```python
from build123d import *

# Parameters (mm, degrees)
SKETCH1_W                  = 20
SKETCH1_H                  = 37.5
SKETCH1_W_2                = 192
SKETCH1_H_2                = 30
BOSS_EXTRUDE1_DEPTH        = 10
F_4_0_209_DIAMETER_HOLE1_D = 5.3086
SKETCH6_W                  = 15
SKETCH6_H                  = 30
BOSS_EXTRUDE2_DEPTH        = 30
BOSS_EXTRUDE3_START        = 30
SKETCH6_3_W                = 100
SKETCH6_3_H                = 30
SKETCH6_3_W_2              = 15
BOSS_EXTRUDE3_DEPTH        = 15
FILLET2_R                  = 7


with BuildPart() as part:
    # Sketch1 → Boss-Extrude1 (new body)
    with BuildSketch(Plane.XY):
        with Locations((-86, 33.75)):
            Rectangle(SKETCH1_W, SKETCH1_H)
        Rectangle(SKETCH1_W_2, SKETCH1_H_2)
        with Locations((-86, -33.75)):
            Rectangle(SKETCH1_W, SKETCH1_H)
        with Locations((86, -33.75)):
            Rectangle(SKETCH1_W, SKETCH1_H)
        with Locations((86, 33.75)):
            Rectangle(SKETCH1_W, SKETCH1_H)
    extrude(amount=BOSS_EXTRUDE1_DEPTH)

    # #4 (0.209) Diameter Hole1 (through all)
    with Locations(Plane.XY.offset(10)):
        with Locations((-86, 42.5), (-86, -42.5), (86, -42.5), (86, 42.5)):
            Hole(F_4_0_209_DIAMETER_HOLE1_D / 2)

    # Sketch6 → Boss-Extrude2 (add)
    with BuildSketch(Plane.XY.offset(10)):
        with Locations((-57.5, 0)):
            Rectangle(SKETCH6_W, SKETCH6_H)
        with Locations((57.5, 0)):
            Rectangle(SKETCH6_W, SKETCH6_H)
    extrude(amount=BOSS_EXTRUDE2_DEPTH)

    # Sketch6<3> → Boss-Extrude3 (add)
    with BuildSketch(Plane.XY.offset(10).offset(BOSS_EXTRUDE3_START)):
        Rectangle(SKETCH6_3_W, SKETCH6_3_H)
        with Locations((-57.5, 0)):
            Rectangle(SKETCH6_3_W_2, SKETCH6_3_H)
        with Locations((57.5, 0)):
            Rectangle(SKETCH6_3_W_2, SKETCH6_3_H)
    extrude(amount=BOSS_EXTRUDE3_DEPTH)

    # Fillet2
    fillet2_edges = [part.edges().sort_by_distance(p)[0] for p in [
        (0, 15, 40),
        (0, -15, 40),
        (0, 15, 55),
        (-65, 0, 55),
        (0, -15, 55),
        (65, 0, 55),
        (-70.5, -15, 10),
        (-70.5, 15, 10),
        (0, -15, 10),
        (70.5, -15, 10),
        (0, 15, 10),
        (70.5, 15, 10),
        (-50, 15, 25),
        (-65, 0, 10),
        (-65, 15, 32.5),
        (-65, -15, 32.5),
        (-50, -15, 25),
        (-50, 0, 10),
        (65, -15, 32.5),
        (65, 15, 32.5),
        (50, 0, 10),
        (50, 15, 25),
        (50, -15, 25),
        (65, 0, 10),
    ]]
    fillet(fillet2_edges, radius=FILLET2_R)


solid = part.part
```
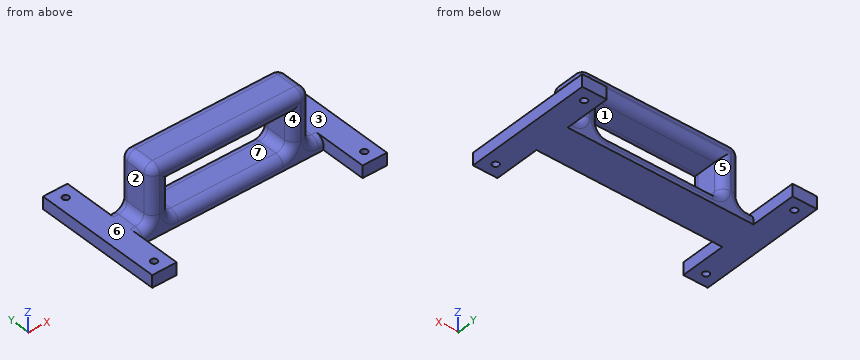
Work out the finished part from the listing and answer in its coordinate system (mm). Face numbers are marked on the shaded views. A direction names the side the tool comes from. Give positions to 0.01 mm unless a question says otherwise; leave off trailing zeros. Order: outer loops, then holes, each group sorted by start corner. A loop starts at its lowest first (then second) coordinate and runs counter-clockwise, first axis right, second up. Notation, with made-up numbers: (27.25, 65.5) - (70.25, 65.5) arc R20 cw to (70.25, 98.5) - close; hole circle Ø7 at (30.5, -28). An arc over 180 degrees is marked (long way). One line per item, written item: value. Start each with the question number.
1. Section A-A, the plane z = 34 is taken. Write down the section's boundary in (x, y).
2. Section C-C, the plane y = -23 is taken. Write down the section's boundary in (x, z), then the cut area to 3 significant figures.
3. Which of the six approach directions +Z, -Z, +X, -X, +Y, -Y give full straight-line access (tool end or side, diameter ignored) to the marked faces 4, 5, 6 and 7?
4. Section B-B, the plane x = -86 is taken. Write down the section's boundary in (y, z).
5. For a pull along Z with two mould halves and no side action, classify the marked faces 1, 2 and 3 as released by +Z, released by -Z, zero draft, split by the parting line, or undercut.
6. Consider line 1 (Y direction, x = 86, z = 5); line 2 (X direction, y = 34.5, z = 6.5); line 3 (X direction, y = 42, z = 3). Determine where each line is inside the solid, lowest interval first.
7. Section D-D, the plane x = -32 is taken. Write down the section's boundary in (y, z).
8. Each of these flat-tipped pins is pushed along its axis until it touches: pin 1 Ø8 at (y, z) = (2, 30) entering from -X; pin 2 Ø6 at (x, y) = (-86, -42.5) entering from +Z; pin 3 Ø17.5 at (y, z) = (-2.5, 33.5) entering from +X. Where does it stop, or does it pass through?
Filled sheet:
1. outline: (-65, -8) arc R7 ccw to (-58, -15) - (-57, -15) arc R7 ccw to (-50, -8) - (-50, 8) arc R7 ccw to (-57, 15) - (-58, 15) arc R7 ccw to (-65, 8) - close; (50, -8) arc R7 ccw to (57, -15) - (58, -15) arc R7 ccw to (65, -8) - (65, 8) arc R7 ccw to (58, 15) - (57, 15) arc R7 ccw to (50, 8) - close
2. outline: (-96, 0) - (-76, 0) - (-76, 10) - (-96, 10) - close; (76, 0) - (96, 0) - (96, 10) - (76, 10) - close
2. area: 400 mm²
3. face 4: -Y
3. face 5: +Y
3. face 6: +Z, -X, +Y, -Y
3. face 7: +Y, -Y
4. outline: (-52.5, 0) - (-45.15, 0) - (-45.15, 10) - (-52.5, 10) - close; (-39.85, 0) - (39.85, 0) - (39.85, 10) - (-39.85, 10) - close; (45.15, 0) - (52.5, 0) - (52.5, 10) - (45.15, 10) - close
5. face 1: undercut
5. face 2: zero draft
5. face 3: released by +Z
6. line 1: -52.5 to -45.15, -39.85 to 39.85, 45.15 to 52.5
6. line 2: -96 to -76, 76 to 96
6. line 3: -96 to -88.61, -83.39 to -76, 76 to 83.39, 88.61 to 96
7. outline: (-15, 0) - (15, 0) - (15, 3) arc R7 ccw to (8, 10) - (-8, 10) arc R7 ccw to (-15, 3) - close; (-15, 47) arc R7 ccw to (-8, 40) - (8, 40) arc R7 ccw to (15, 47) - (15, 48) arc R7 ccw to (8, 55) - (-8, 55) arc R7 ccw to (-15, 48) - close
8. pin 1: x = -65
8. pin 2: z = 10
8. pin 3: x = 65
